Work out the finished part from the listing and answer in its coordinate system (mm). Face numbers are marked on the shaded views. A direction names the side the tool comes from. Coordinates: 2 decimals unless noted, no trailing zeros. Order: outer loops, then holes, each group sorted by start corner. A loop starts at its lowest first (then second) coordinate and runs counter-clockwise, first axis right, second up. Notation, with made-up numbers: (45.5, -4.5) - (89.5, -4.5) arc R14 ccw to (89.5, 22.5) - close; hole circle Ø10 at (20.5, -4). An arc over 180 degrees is marked (long way). Answer as a JSON object with one key per item and string values. Group by question number.
1) Find the intervals of material crossed by line 1 along Y through (x, z) = (0, 7); line 2 along Y through (x, z) = (15, 47.5); line 3 along Y through (x, z) = (-46, 47), in increasing order.
2) The mould has two halves that part along Z. Classify the marked faces 1, 2, 3 and 4: released by +Z, released by -Z, zero draft, split by the parting line, or undercut.
3) Each of these flat-tipped pins is pushed along its axis until it touches: P1, Ø6, axis at x = -9.5, z = 15, coming from the -Y side; P2, Ø5, axis at y = 13.5, z = 14, coming from the +X side; P3, Ø4, axis at y = 12.5, z = 8, coming from the -X side; P4, Ø12, axis at x = 30.5, z = 34.5, coming from the +Y side. Where does it stop, or does it pass through?
4) Section B-B (x = 0) is taken. Give the vertices of the cut face in (y, z).
5) Section A-A (y = -25) is taken. Give the vertices of the cut face in (x, z), plus the area to 3 significant figures.
6) A tool of negligible diameter and unlimited length cuts with its end or side. For the marked faces 5, 6, 7 and 8, from which of +Z, -Z, +X, -X, +Y, -Y can it reach the whole face along a straight path? Write none if from no direction.
7) Section C-C (z = 45) is taken. Give the vertices of the cut face in (x, y), plus the area to 3 significant figures.
8) Section D-D (y = 18) is taken. Give the vertices of the cut face in (x, z), plus the area to 3 significant figures.
from build123d import *

# Parameters (mm, degrees)
F0_W      = 78
F0_H      = 70
F1_DEPTH  = 10
F3_DEPTH  = 70
F5_D      = 5.2
F6_W      = 100
F6_H      = 30
F7_DEPTH  = 40
F8_W      = 100
F8_H      = 7
F9_DEPTH  = 15
F11_DEPTH = 50.001
F12_R     = 2
F13_W     = 0.5
F13_H     = 7.4945365116
F14_DEPTH = 1
F15_D     = 2.5
F15_DEPTH = 10
F15_TIP   = 0.7510757738


with BuildPart() as f1:
    # F0 (on Top) → F1 (new body)
    with BuildSketch(Plane.XY):
        Rectangle(F0_W, F0_H)
    extrude(amount=F1_DEPTH)

    # F2 (on face) → F3 (cut)
    with BuildSketch(Plane.XZ.offset(35)):
        Polygon((-39, 10), (-39, 0), (-29, 10), align=None)
        Polygon((29, 10), (39, 0), (39, 10), align=None)
    extrude(amount=-F3_DEPTH, mode=Mode.SUBTRACT)

    # F5 (through all)
    with Locations(Plane.XY.offset(10)):
        with Locations((0, 25), (0, -25)):
            Hole(F5_D / 2)

    # F6 (on face) → F7 (join)
    with BuildSketch(Plane.XY.offset(10)):
        Rectangle(F6_W, F6_H)
    extrude(amount=F7_DEPTH)

    # F8 (on face) → F9 (cut)
    with BuildSketch(Plane.XY.offset(50)):
        Rectangle(F8_W, F8_H)
    extrude(amount=-F9_DEPTH, mode=Mode.SUBTRACT)

    # F10 (on face) → F11 (cut, through all)
    with BuildSketch(Plane(origin=(0, 15, 0), x_dir=(-1, 0, 0), z_dir=(0, 1, 0))):
        Polygon((-50, 10), (-29, 10), (-30.3908418864, 10.3), (-50, 10.3), align=None)
        Polygon((30.3908418864, 10.3), (29, 10), (50, 10), (50, 10.3), align=None)
    extrude(amount=-F11_DEPTH, mode=Mode.SUBTRACT)

    # F12
    f12_edges = [f1.edges().sort_by_distance(p)[0] for p in [
        (29, -25, 10),
        (29, 25, 10),
        (34, 35, 5),
        (39, 0, 0),
        (34, -35, 5),
        (0, 35, 10),
        (0, -35, 10),
        (0, -15, 50),
        (0, -3.5, 50),
        (0, 3.5, 50),
        (0, 15, 50),
        (50, 15, 30.15),
        (50, -15, 30.15),
        (50, 0, 10.3),
        (-29, -25, 10),
        (-50, -15, 30.15),
        (-50, 15, 30.15),
        (-50, 0, 10.3),
        (-39, 0, 0),
        (-34, -35, 5),
        (-34, 35, 5),
    ]]
    fillet(f12_edges, radius=F12_R)

    # F13 (on face) → F14 (cut)
    with BuildSketch(Plane.XY.offset(50)):
        with Locations((27.87883, 9.2527317442)):
            Rectangle(F13_W, F13_H)
        with Locations((26.87883, 9.2527317442)):
            Rectangle(F13_W, F13_H)
        with Locations((25.87883, 9.2527317442)):
            Rectangle(F13_W, F13_H)
        with Locations((24.87883, 9.2527317442)):
            Rectangle(F13_W, F13_H)
        with Locations((23.87883, 9.2527317442)):
            Rectangle(F13_W, F13_H)
        with Locations((22.87883, 9.2527317442)):
            Rectangle(F13_W, F13_H)
        with Locations((27.87883, -9.2527317442)):
            Rectangle(F13_W, F13_H)
        with Locations((26.87883, -9.2527317442)):
            Rectangle(F13_W, F13_H)
        with Locations((25.87883, -9.2527317442)):
            Rectangle(F13_W, F13_H)
        with Locations((24.87883, -9.2527317442)):
            Rectangle(F13_W, F13_H)
        with Locations((23.87883, -9.2527317442)):
            Rectangle(F13_W, F13_H)
        with Locations((22.87883, -9.2527317442)):
            Rectangle(F13_W, F13_H)
    extrude(amount=-F14_DEPTH, mode=Mode.SUBTRACT)

    # F15
    with Locations(Plane.XY.offset(50)):
        with Locations((15, 9.253), (15, -9.253)):
            Hole(F15_D / 2, depth=F15_DEPTH)
            with Locations((0, 0, -(F15_DEPTH + F15_TIP / 2))):  # 118° drill point
                Cone(0, F15_D / 2, F15_TIP, mode=Mode.SUBTRACT)


solid = f1.part
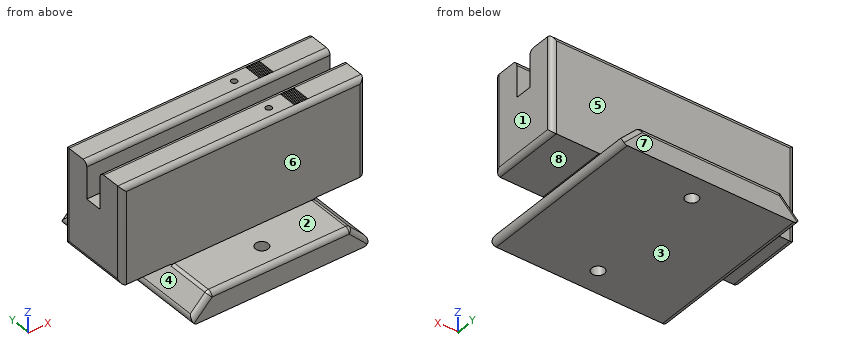
Report:
{
 "1": {"line 1": "y = -35 to -27.6, -22.4 to 22.4, 27.6 to 35", "line 2": "y = -15 to -10.5, -8 to -3.5, 3.5 to 8, 10.5 to 15", "line 3": "y = -15 to -3.5, 3.5 to 15"},
 "2": {"face 1": "zero draft", "face 2": "released by +Z", "face 3": "released by -Z", "face 4": "undercut"},
 "3": {"P1": "stops at y = -15", "P2": "stops at x = 50", "P3": "stops at x = -33", "P4": "stops at y = 15"},
 "4": {"outline": "(-35, 0) - (-27.6, 0) - (-27.6, 10) - (-33, 10) arc R2 ccw to (-35, 8) - close; (-22.4, 0) - (22.4, 0) - (22.4, 10) - (15, 10) - (15, 48) arc R2 ccw to (13, 50) - (5.5, 50) arc R2 ccw to (3.5, 48) - (3.5, 35) - (-3.5, 35) - (-3.5, 48) arc R2 ccw to (-5.5, 50) - (-13, 50) arc R2 ccw to (-15, 48) - (-15, 10) - (-22.4, 10) - close; (27.6, 0) - (35, 0) - (35, 8) arc R2 ccw to (33, 10) - (27.6, 10) - close"},
 "5": {"outline": "(-35.59, 3.41) arc R2 ccw to (-34.17, 0) - (-2.6, 0) - (-2.6, 10) - (-28.17, 10) arc R2 ccw to (-29.59, 9.41) - close; (2.6, 0) - (34.17, 0) arc R2 ccw to (35.59, 3.41) - (29.59, 9.41) arc R2 ccw to (28.17, 10) - (2.6, 10) - close", "area": "618 mm²"},
 "6": {"face 5": "+Z, +X, -X, +Y", "face 6": "+Z, +X, -X, -Y", "face 7": "+Z, -Z, +X, -X, +Y", "face 8": "+X, +Y, -Y"},
 "7": {"outline": "(-50, -13) arc R2 ccw to (-48, -15) - (48, -15) arc R2 ccw to (50, -13) - (50, -3.5) - (-50, -3.5) - close; (-50, 3.5) - (50, 3.5) - (50, 13) arc R2 ccw to (48, 15) - (-48, 15) arc R2 ccw to (-50, 13) - close; hole circle Ø2.5 at (15, -9.25); hole circle Ø2.5 at (15, 9.25)", "area": "2,290 mm²"},
 "8": {"outline": "(-35.59, 3.41) arc R2 ccw to (-34.17, 0) - (34.17, 0) arc R2 ccw to (35.59, 3.41) - (29.59, 9.41) arc R2 ccw to (28.17, 10) - (-29, 10) - close", "area": "670 mm²"}
}
